Read the model definition and answer for the solid it produces. Units are mm, in the model's axes. Face numbers are marked on the shaded views. Round coordinates to 2 decimals unless told otherwise and drop trailing zeros. Order: outer loops, then holes, each group sorted by start corner. A loop starts at its lowest first (then second) coordinate and runs counter-clockwise, first axis right, second up. Notation, with made-up numbers: (8, 80.5) - (53, 80.5) arc R26 ccw to (53, 100.5) - close; hole circle Ø11 at (-9, -16). An arc over 180 degrees is marked (long way). One line per question, with ' | ' between items. Start each with the question number.
1) The part is cut by section C-C, the plane y = 15.24. Give the vertices of the cut face in (x, z), plus the area to 3 significant figures.
2) The part is cut by section B-B, the plane x = 29.21. Give the vertices of the cut face in (y, z), plus the area to 3 significant figures.
3) The mould has two halves that part along X. Classify the marked faces 1, 2 and 3: pulls with the +X half, pulls with the -X half, needs draft (parallel to the pull), parting line crosses it, or undercut.
4) Straight lines are drawn through the part: line 1 (Y direction, x = 8.89, z = -8.75); line 2 (Y direction, x = 19.05, z = -4); line 3 (X direction, y = 15.5, z = -9.25). For each, find the intervals that lie inside material, in ascending order. Write a range as from..to.
5) The part is cut by section A-A, the plane y = 36.83. Give the vertices of the cut face in (x, z), plus the area to 3 significant figures.
6) A flat-ended cylindrical pin translates along its axis: pin 1 (11 mm diameter, centred on x = 8.89, y = 36.83, fed in from -Z). Find the tip coordinate at first contact, or state that the pin passes through.
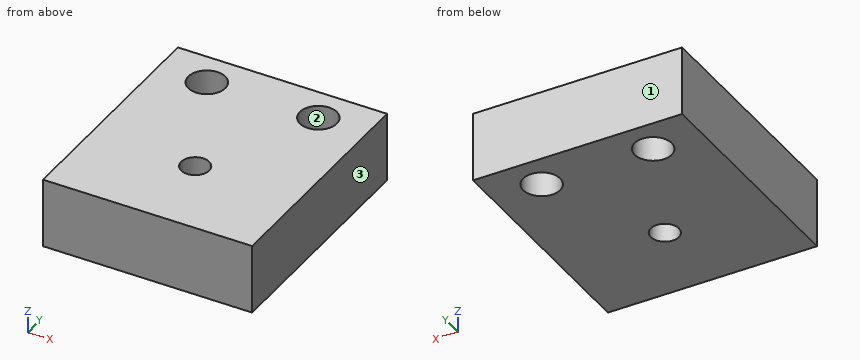
from build123d import *

# Parameters (mm, degrees)
SKETCH1_W                        = 38.1
SKETCH1_H                        = 43.18
BOSS_EXTRUDE1_DEPTH              = 12.7
F_17_64_0_26563_DIAMETER_HOLE1_D = 6.747002
F_1_4_20_TAPPED_HOLE1_D          = 5.1054
F_1_4_20_TAPPED_HOLE1_DEPTH      = 12.7


with BuildPart() as part:
    # Sketch1 → Boss-Extrude1 (new body)
    with BuildSketch(Plane.XY):
        with Locations((19.05, 21.59)):
            Rectangle(SKETCH1_W, SKETCH1_H)
    extrude(amount=-BOSS_EXTRUDE1_DEPTH)

    # 17/64 (0.26563) Diameter Hole1 (through all)
    with Locations(Plane(origin=(29.21, 36.83, 0), x_dir=(1, 0, 0), z_dir=(0, 0, 1))):
        with Locations((0, 0), (-20.32, 0)):
            Hole(F_17_64_0_26563_DIAMETER_HOLE1_D / 2)

    # 1/4-20 Tapped Hole1
    with Locations(Plane.XY):
        with Locations((19.05, 15.24)):
            Hole(F_1_4_20_TAPPED_HOLE1_D / 2, depth=F_1_4_20_TAPPED_HOLE1_DEPTH)


solid = part.part
Values:
1) outline: (0, -12.7) - (16.5, -12.7) - (16.5, 0) - (0, 0) - close; (21.6, -12.7) - (38.1, -12.7) - (38.1, 0) - (21.6, 0) - close | area: 419 mm^2
2) outline: (0, -12.7) - (33.46, -12.7) - (33.46, 0) - (0, 0) - close; (40.2, -12.7) - (43.18, -12.7) - (43.18, 0) - (40.2, 0) - close | area: 463 mm^2
3) face 1: needs draft | face 2: undercut | face 3: pulls with the +X half
4) line 1: y = 0..33.46, 40.2..43.18 | line 2: y = 0..12.69, 17.79..43.18 | line 3: x = 0..16.51, 21.59..38.1
5) outline: (0, -12.7) - (5.52, -12.7) - (5.52, 0) - (0, 0) - close; (12.26, -12.7) - (25.84, -12.7) - (25.84, 0) - (12.26, 0) - close; (32.58, -12.7) - (38.1, -12.7) - (38.1, 0) - (32.58, 0) - close | area: 312 mm^2
6) pin 1: stops at z = -12.7
